Geometry: final body of the model. Coordinates: model frame, mm. Give positions to 0.01 mm unless a question says otherwise; leave off trailing zeros. Write each loop counter-clockwise with the first axis right and the second up, starting at its lowest first coordinate (ties: lowest second). Pieces come first, ordered by that corner, then holes. Notation, with made-up numbers: (-4.5, -15.5) - (53.5, -15.5) arc R17 cw to (53.5, 4.5) - close; hole circle Ø3 at (-34, 17). An arc over 180 degrees is marked (long way). Return JSON: item names as keys, results as strings.
Autodesk Inventor part; units mm, degrees
ref_plane "1_XY" through (2, 0, 0) normal (1, 0, 0) x (0, 0, -1)
ref_plane "1_YZ" through (2, 0, 0) normal (0, 0, -1) x (0, 1, 0)
ref_plane "1_ZX" through (2, 0, 0) normal (0, 1, 0) x (1, 0, 0)
sketch "Sketch_1" plane through (0, 0, 0) normal (0, 0, 1) x (1, 0, 0)
  line L0 (4, 0) -> (0, 0)
  line L1 (0, 10.85) -> (0, 10.04)
  arc A0 (0, 10.04) -> (0.075, 9.965) centre (0.075, 10.04) ccw
  line L2 (0.075, 9.965) -> (1.3567, 9.965)
  arc A1 (2.6433, 9.965) -> (1.3567, 9.965) centre (2, 9.5) ccw
  line L3 (2.6433, 9.965) -> (3.925, 9.965)
  arc A2 (3.925, 9.965) -> (4, 10.04) centre (3.925, 10.04) ccw
  line L4 (4, 10.04) -> (4, 10.85)
  arc A3 (4, 10.85) -> (3.85, 11) centre (3.85, 10.85) ccw
  line L5 (3.85, 11) -> (0.15, 11)
  arc A4 (0.15, 11) -> (0, 10.85) centre (0.15, 10.85) ccw
revolve "Revolution1" add sketch "Sketch_1" angle 360 about axis through (4, 0, 0) along (1, 0, 0)
ref_plane "1_XY" through (2, 0, 0) normal (1, 0, 0) x (0, 0, -1)
ref_plane "1_YZ" through (2, 0, 0) normal (0, 0, -1) x (0, 1, 0)
ref_plane "1_ZX" through (2, 0, 0) normal (0, 1, 0) x (1, 0, 0)
properties part number "A-2216_or"
Q1. Section query D-D, the plane x = 2.1. Return the cut outline in (y, z).
Answer key:
{"outline": "circle Ø22 at (0, 0); hole circle Ø20.57 at (0, 0)"}
Q2. Mould query, pull axis Z, two halves, no side actions, for faces 1 (the cylindrical face through (3.293, 9.505, 2.993)), 2 (the flat face through (0, 10, -3)), 3 (the cylindrical face through (1.97, -2.38, 10.74)). Classes: pulls with the +Z half, pulls with the -Z half, needs draft (parallel to the pull), parting line crosses it, or undercut.
Answer key:
{"face 1": "undercut", "face 2": "needs draft", "face 3": "parting line crosses it"}
Q3. Material intervals for probe 1 along Z at (x, y) = (3.5, 0) (3 decimals); probe 2 along Z at (x, y) = (1.65, 0.75); probe 3 along Y at (x, z) = (3.35, 5.5), sorted ascending. Write a range as [from, to].
Answer key:
{"probe 1": "z = [-11, -9.965], [9.965, 11]", "probe 2": "z = [-10.97, -10.18], [10.18, 10.97]", "probe 3": "y = [-9.53, -8.31], [8.31, 9.53]"}
Q4. Section query A-A, the plane z = 0. Return the cut outline in (x, y) (3 decimals).
Answer key:
{"outline": "(0, -10.85) arc R0.15 ccw to (0.15, -11) - (3.85, -11) arc R0.15 ccw to (4, -10.85) - (4, -10.04) arc R0.075 ccw to (3.925, -9.965) - (2.643, -9.965) arc R0.794 cw to (1.357, -9.965) - (0.075, -9.965) arc R0.075 ccw to (0, -10.04) - close; (0, 10.04) arc R0.075 ccw to (0.075, 9.965) - (1.357, 9.965) arc R0.794 cw to (2.643, 9.965) - (3.925, 9.965) arc R0.075 ccw to (4, 10.04) - (4, 10.85) arc R0.15 ccw to (3.85, 11) - (0.15, 11) arc R0.15 ccw to (0, 10.85) - close"}
Q5. Pin query (flat end, axial travel): P1, Ø5, axis at y = 0, z = 6, coming from the -X side. Return the tip coordinate at first contact, or that it passes through.
Answer key:
{"P1": "passes through"}
Q6. Section query C-C, the plane x = 0.6. Return the cut outline in (y, z) (3 decimals).
Answer key:
{"outline": "circle Ø22 at (0, 0); hole circle Ø19.93 at (0, 0)"}
